Verification items for the finished model (mm, model axes). A direction names the side the tool comes from. Round coordinates to 2 decimals unless told otherwise and drop trailing zeros. Loops run counter-clockwise (first coordinate to the right, second up) from the corner with the lowest first, then second, coordinate; pieces in that order, holes last. Notation, with made-up numbers: M -10.75,72 L 45.25,72 A29 cw 45.25,107 Z; hole C -8,-12 d1. An arc over 180 degrees is marked long. One line per item, written item: value.
Autodesk Inventor part; units mm, degrees
ref_plane "YZ Plane" through (0, 0, 0) normal (1, 0, 0) x (0, 1, 0)
ref_plane "XZ Plane" through (0, 0, 0) normal (0, 1, 0) x (-1, 0, 0)
ref_plane "XY Plane" through (0, 0, 0) normal (0, 0, 1) x (1, 0, 0)
sketch "Esquisse1" plane through (0, 0, 0) normal (0, 0, 1) x (1, 0, 0)
  circle A0 centre (0, 0) radius 18.4
  circle A1 centre (0, -7) radius 6
  circle A2 centre (15.5, 0) radius 1.25
  circle A3 centre (7.75, -13.4234) radius 1.25
  circle A4 centre (-7.75, -13.4234) radius 1.25
  circle A5 centre (-15.5, 0) radius 1.25
  circle A6 centre (-7.75, 13.4234) radius 1.25
  circle A7 centre (7.75, 13.4234) radius 1.25
  circle A8 centre (0, 15.5) radius 1.9
  circle A9 centre (-13.4234, -7.75) radius 1.9
  circle A10 centre (13.4234, -7.75) radius 1.9
  arc A11 (9.2253, -8.2857) -> (-9.2253, -8.2857) centre (0, 0) ccw
  spline S0 degree 3 poles (9.2254, -8.2857) (9.1718, -8.3454) (9.1113, -8.4012) (8.9929, -8.4831) (8.9346, -8.5143) (8.8333, -8.5456) (8.791, -8.5527) (8.7144, -8.5502) (8.6808, -8.5434) (8.6178, -8.5166) (8.59, -8.4975) (8.5381, -8.4462) (8.5162, -8.4136) (8.4741, -8.3274) (8.4589, -8.2705) (8.4364, -8.1241) (8.4381, -8.0284) (8.4482, -7.9376) knots -0.133179 -0.133179 -0.133179 -0.133179 -0.109147 -0.109147 -0.089905 -0.089905 -0.077133 -0.077133 -0.066705 -0.066705 -0.05641 -0.05641 -0.044636 -0.044636 -0.027428 -0.027428 0 0 0 0
  arc A12 (8.4481, -7.9376) -> (-8.4481, -7.9376) centre (0, -7) ccw
  spline S1 degree 3 poles (-8.4482, -7.9376) (-8.4382, -8.0273) (-8.4365, -8.1217) (-8.4582, -8.2676) (-8.4733, -8.3251) (-8.5152, -8.412) (-8.537, -8.4449) (-8.5887, -8.4966) (-8.6164, -8.5158) (-8.6792, -8.543) (-8.7127, -8.5499) (-8.7891, -8.5529) (-8.8312, -8.546) (-8.932, -8.5155) (-8.99, -8.4848) (-9.1093, -8.403) (-9.1709, -8.3463) (-9.2254, -8.2857) knots -0.133396 -0.133396 -0.133396 -0.133396 -0.106249 -0.106249 -0.088887 -0.088887 -0.077046 -0.077046 -0.066737 -0.066737 -0.056304 -0.056304 -0.043575 -0.043575 -0.024448 -0.024448 0 0 0 0
  line L0 (-21, 21) -> (21, 21)
  line L1 (21, 21) -> (21, -25)
  line L2 (21, -25) -> (-21, -25)
  line L3 (-21, -25) -> (-21, 21)
  circle A13 centre (-7.75, 13.4234) radius 1.75
  circle A14 centre (-15.5, 0) radius 1.75
  circle A15 centre (7.75, 13.4234) radius 1.75
  circle A16 centre (15.5, 0) radius 1.75
  circle A17 centre (-7.75, -13.4234) radius 1.75
  circle A18 centre (7.75, -13.4234) radius 1.75
  circle A19 centre (-7.75, 13.4234) radius 1.75
  circle A20 centre (7.75, 13.4234) radius 1.75
  circle A21 centre (15.5, 0) radius 1.75
  circle A22 centre (7.75, -13.4234) radius 1.75
  circle A23 centre (-7.75, -13.4234) radius 1.75
  circle A24 centre (-15.5, 0) radius 1.75
  circle A25 centre (0, -7) radius 6
extrude "Extrusion1" add sketch "Esquisse1" along normal blind 2 contours A0 | A8 | A9 | A10 | S0 A12 S1 A11 | L0 L1 L2 L3
sketch "Esquisse2" plane through (0, 0, 0) normal (0, 0, -1) x (-1, 0, 0)
  line L0 (-21, 21) -> (-21, -25)
  line L1 (21, -25) -> (-21, -25)
  line L2 (-21, -25) -> (-21, -23)
  line L3 (-21, -23) -> (21, -23)
  line L4 (21, -23) -> (21, -25)
  point P0 (0, 0)
  dimension "d7" = 2
extrude "Extrusion2" add sketch "Esquisse2" along normal blind 50
sketch "Esquisse3" plane through (-21, -25, 2) normal (0, -1, 0) x (1, 0, 0)
  line L0 (0, 0) -> (0, -52)
  line L1 (42, -52) -> (0, -52)
  point P0 (21, -2)
  point P1 (5, -47)
  point P2 (5, -27)
  point P3 (5, -7)
  point P4 (37, -47)
  point P5 (37, -27)
  point P6 (37, -7)
  dimension "d10" = 5
  dimension "d11" = 5
  dimension "d12" = 52
  dimension "d15" = 20
  dimension "d18" = 32
hole "Perçage1" at (-16, -25, -45) at (-16, -25, -25) at (-16, -25, -5) at (16, -25, -45) at (16, -25, -25) at (16, -25, -5) direction (0, 1, 0) diameter 3 end through all
properties part number "support_moteur"
(1) Mould release check, pull along X, two halves, no side actions. Record for faces 1 (the face through (0, -25, -24)), 2 (the face through (21, -24, -12)), 3 (the face through (-16.07, -23.99, -43.5)): +X half, -X half, draft (parallel to the pull), parting line (faces both ways), or undercut.
Completed:
face 1: draft
face 2: +X half
face 3: undercut
(2) Depth check by flat-ended pin: pin 1 Ø5.5 at (x, y) = (15.5, 0) entering from -Z; pin 2 Ø2 at (x, y) = (-7.75, -13.42) entering from -Z; pin 3 Ø2 at (x, z) = (13.5, -31) entering from +Y. Enter the tip coordinate at first touch or a pass-through.
Completed:
pin 1: stops at z = 0
pin 2: passes through
pin 3: stops at y = -23
(3) Sectioned sample at C-C on y = -7. Enter the section's corners in (x, z).
Completed:
outline: M -21,0 L -6,0 L -6,2 L -21,2 Z; M 6,0 L 21,0 L 21,2 L 6,2 Z
(4) Thickness scan on L1, parallel to Z at x = 16, y = -23.9; L2, parallel to X at y = -24.2, z = -45; L3, parallel to Y at x = 7.75, z = 0.5. Record the ranges inside material, lowest first. Write a range as from..to.
Completed:
L1: z = -50..-46.5, -43.5..-26.5, -23.5..-6.5, -3.5..2
L2: x = -21..-17.5, -14.5..14.5, 17.5..21
L3: y = -25..-15.17, -11.67..11.67, 15.17..21
(5) Sectioned sample at B-B on z = -45. Enter the section's corners in (x, y).
Completed:
outline: M -21,-25 L -17.5,-25 L -17.5,-23 L -21,-23 Z; M -14.5,-25 L 14.5,-25 L 14.5,-23 L -14.5,-23 Z; M 17.5,-25 L 21,-25 L 21,-23 L 17.5,-23 Z
(6) Sectioned sample at D-D on x = -16. Enter the section's corners in (y, z), and give its area (3 significant figures).
Completed:
outline: M -25,-50 L -23,-50 L -23,-46.5 L -25,-46.5 Z; M -25,-43.5 L -23,-43.5 L -23,-26.5 L -25,-26.5 Z; M -25,-23.5 L -23,-23.5 L -23,-6.5 L -25,-6.5 Z; M -25,-3.5 L -23,-3.5 L -23,0 L -1.68,0 L -1.68,2 L -25,2 Z; M 1.68,0 L 21,0 L 21,2 L 1.68,2 Z
area: 167 mm^2
(7) Sectioned sample at A-A on y = 0. Enter the section's corners in (x, z), and give its area (3 significant figures).
Completed:
outline: M -21,0 L -17.25,0 L -17.25,2 L -21,2 Z; M -13.75,0 L 13.75,0 L 13.75,2 L -13.75,2 Z; M 17.25,0 L 21,0 L 21,2 L 17.25,2 Z
area: 70.0 mm^2
(8) Tool access check on faces 4 (the face through (0, -23, -25)), 5 (the face through (15.55, -23.99, -6.43)). Record the directions out of +Z, -Z, +X, -X, +Y, -Y that give a thin tool (end or side, any length) a straight path to the whole face; none if there is none.
Completed:
face 4: -Z, +X, -X, +Y
face 5: +Y, -Y
